Read the model definition and answer for the solid it produces. Units are mm, in the model's axes. A direction names the side the tool comes from. Give positions to 0.01 mm unless a question says otherwise; leave off trailing zeros. Loops run counter-clockwise (first coordinate to the right, second up) from the corner with the lowest first, then second, coordinate; pieces in that order, holes last. Notation, with made-up numbers: (58, 87) - (105, 87) arc R6 ccw to (105, 94) - close; hole circle Ø8 at (35, -12.5). An arc over 180 degrees is marked (long way). Write item = value, one per line. Start each with the question number.
from build123d import *

# Parameters (mm, degrees)
F0_W     = 1333.5
F0_H     = 1524
F0_W_2   = 34.925
F0_H_2   = 63.5
F0_W_3   = 63.5
F0_H_3   = 15.875
F0_W_4   = 15.875
F0_H_4   = 15
F0_H_5   = 95.25
F0_W_5   = 184.15
F0_H_6   = 101.6
F1_DEPTH = 12.7
F2_START = 12.7
F2_DEPTH = 355.6


with BuildPart() as f1:
    # F0 (on Front) → F1 (new body)
    with BuildSketch(Plane.XZ):
        with Locations((666.75, 762)):
            Rectangle(F0_W, F0_H)
        with Locations((166.6875, 39.6875)):
            Rectangle(F0_W_2, F0_H_2, mode=Mode.SUBTRACT)
        with Locations((166.6875, 357.1875)):
            Rectangle(F0_W_2, F0_H_2, mode=Mode.SUBTRACT)
        with Locations((627.0625, 93.6625)):
            Rectangle(F0_W_3, F0_H_3, mode=Mode.SUBTRACT)
        with Locations((627.0625, 279.4)):
            Rectangle(F0_W_3, F0_H_3, mode=Mode.SUBTRACT)
        with Locations((166.6875, 436.5625)):
            Rectangle(F0_W_2, F0_H_2, mode=Mode.SUBTRACT)
        with Locations((92.075, 728.6625)):
            Rectangle(F0_W_4, F0_H_2, mode=Mode.SUBTRACT)
        with Locations((241.3, 728.6625)):
            Rectangle(F0_W_4, F0_H_2, mode=Mode.SUBTRACT)
        with Locations((627.0625, 514.35)):
            Rectangle(F0_W_3, F0_H_3, mode=Mode.SUBTRACT)
        with Locations((627.0625, 650.875)):
            Rectangle(F0_W_3, F0_H_3, mode=Mode.SUBTRACT)
        with Locations((847.725, 39.6875)):
            Rectangle(F0_W_2, F0_H_2, mode=Mode.SUBTRACT)
        with Locations((960.4375, 193.2375)):
            Rectangle(F0_W_3, F0_H_4, mode=Mode.SUBTRACT)
        with Locations((1293.8125, 93.6625)):
            Rectangle(F0_W_3, F0_H_3, mode=Mode.SUBTRACT)
        with Locations((1293.8125, 279.4)):
            Rectangle(F0_W_3, F0_H_3, mode=Mode.SUBTRACT)
        with Locations((847.725, 436.5625)):
            Rectangle(F0_W_2, F0_H_2, mode=Mode.SUBTRACT)
        with Locations((960.4375, 577.85)):
            Rectangle(F0_W_3, F0_H_3, mode=Mode.SUBTRACT)
        with Locations((1293.8125, 514.35)):
            Rectangle(F0_W_3, F0_H_3, mode=Mode.SUBTRACT)
        with Locations((1293.8125, 650.875)):
            Rectangle(F0_W_3, F0_H_3, mode=Mode.SUBTRACT)
        with Locations((25.4, 808.0375)):
            Rectangle(F0_W_2, F0_H_2, mode=Mode.SUBTRACT)
        with Locations((214.3125, 1084.2625)):
            Rectangle(F0_W_4, F0_H_5, mode=Mode.SUBTRACT)
        with Locations((403.225, 808.0375)):
            Rectangle(F0_W_2, F0_H_2, mode=Mode.SUBTRACT)
        with Locations((188.9125, 1179.5125)):
            Rectangle(F0_W_4, F0_H_2, mode=Mode.SUBTRACT)
        with Locations((117.475, 1484.3125)):
            Rectangle(F0_W_4, F0_H_2, mode=Mode.SUBTRACT)
        with Locations((260.35, 1484.3125)):
            Rectangle(F0_W_4, F0_H_2, mode=Mode.SUBTRACT)
        with Locations((617.5375, 1244.6)):
            Rectangle(F0_W_3, F0_H_3, mode=Mode.SUBTRACT)
        with Locations((477.8375, 1406.525)):
            Rectangle(F0_W_5, F0_H_3, mode=Mode.SUBTRACT)
        with Locations((1109.6625, 1081.0875)):
            Rectangle(F0_W_4, F0_H_6, mode=Mode.SUBTRACT)
        with Locations((915.9875, 1419.225)):
            Rectangle(F0_W_3, F0_H_3, mode=Mode.SUBTRACT)
        with Locations((1144.5875, 1179.5125)):
            Rectangle(F0_W_4, F0_H_2, mode=Mode.SUBTRACT)
        with Locations((1144.5875, 1484.3125)):
            Rectangle(F0_W_4, F0_H_2, mode=Mode.SUBTRACT)
        with Locations((477.8375, 1406.525)):
            Rectangle(F0_W_5, F0_H_3)
        with Locations((166.6875, 39.6875)):
            Rectangle(F0_W_2, F0_H_2)
        with Locations((847.725, 39.6875)):
            Rectangle(F0_W_2, F0_H_2)
        with Locations((166.6875, 357.1875)):
            Rectangle(F0_W_2, F0_H_2)
        with Locations((166.6875, 436.5625)):
            Rectangle(F0_W_2, F0_H_2)
        with Locations((847.725, 436.5625)):
            Rectangle(F0_W_2, F0_H_2)
        with Locations((403.225, 808.0375)):
            Rectangle(F0_W_2, F0_H_2)
        with Locations((25.4, 808.0375)):
            Rectangle(F0_W_2, F0_H_2)
        with Locations((1109.6625, 1081.0875)):
            Rectangle(F0_W_4, F0_H_6)
        with Locations((214.3125, 1084.2625)):
            Rectangle(F0_W_4, F0_H_5)
        with Locations((627.0625, 93.6625)):
            Rectangle(F0_W_3, F0_H_3)
        with Locations((627.0625, 279.4)):
            Rectangle(F0_W_3, F0_H_3)
        with Locations((1293.8125, 93.6625)):
            Rectangle(F0_W_3, F0_H_3)
        with Locations((1293.8125, 279.4)):
            Rectangle(F0_W_3, F0_H_3)
        with Locations((627.0625, 514.35)):
            Rectangle(F0_W_3, F0_H_3)
        with Locations((960.4375, 577.85)):
            Rectangle(F0_W_3, F0_H_3)
        with Locations((1293.8125, 514.35)):
            Rectangle(F0_W_3, F0_H_3)
        with Locations((1293.8125, 650.875)):
            Rectangle(F0_W_3, F0_H_3)
        with Locations((627.0625, 650.875)):
            Rectangle(F0_W_3, F0_H_3)
        with Locations((92.075, 728.6625)):
            Rectangle(F0_W_4, F0_H_2)
        with Locations((241.3, 728.6625)):
            Rectangle(F0_W_4, F0_H_2)
        with Locations((188.9125, 1179.5125)):
            Rectangle(F0_W_4, F0_H_2)
        with Locations((117.475, 1484.3125)):
            Rectangle(F0_W_4, F0_H_2)
        with Locations((260.35, 1484.3125)):
            Rectangle(F0_W_4, F0_H_2)
        with Locations((617.5375, 1244.6)):
            Rectangle(F0_W_3, F0_H_3)
        with Locations((915.9875, 1419.225)):
            Rectangle(F0_W_3, F0_H_3)
        with Locations((1144.5875, 1484.3125)):
            Rectangle(F0_W_4, F0_H_2)
        with Locations((1144.5875, 1179.5125)):
            Rectangle(F0_W_4, F0_H_2)
        with Locations((960.4375, 193.2375)):
            Rectangle(F0_W_3, F0_H_4)
    extrude(amount=F1_DEPTH)

    # F0 (on Front) → F2 (join)
    with BuildSketch(Plane.XZ.offset(F2_START)):
        with Locations((1144.5875, 1484.3125)):
            Rectangle(F0_W_4, F0_H_2)
        with Locations((1144.5875, 1179.5125)):
            Rectangle(F0_W_4, F0_H_2)
        with Locations((1109.6625, 1081.0875)):
            Rectangle(F0_W_4, F0_H_6)
        with Locations((915.9875, 1419.225)):
            Rectangle(F0_W_3, F0_H_3)
        with Locations((617.5375, 1244.6)):
            Rectangle(F0_W_3, F0_H_3)
        with Locations((188.9125, 1179.5125)):
            Rectangle(F0_W_4, F0_H_2)
        with Locations((260.35, 1484.3125)):
            Rectangle(F0_W_4, F0_H_2)
        with Locations((117.475, 1484.3125)):
            Rectangle(F0_W_4, F0_H_2)
        with Locations((25.4, 808.0375)):
            Rectangle(F0_W_2, F0_H_2)
        with Locations((214.3125, 1084.2625)):
            Rectangle(F0_W_4, F0_H_5)
        with Locations((403.225, 808.0375)):
            Rectangle(F0_W_2, F0_H_2)
        with Locations((241.3, 728.6625)):
            Rectangle(F0_W_4, F0_H_2)
        with Locations((92.075, 728.6625)):
            Rectangle(F0_W_4, F0_H_2)
        with Locations((166.6875, 436.5625)):
            Rectangle(F0_W_2, F0_H_2)
        with Locations((627.0625, 514.35)):
            Rectangle(F0_W_3, F0_H_3)
        with Locations((627.0625, 650.875)):
            Rectangle(F0_W_3, F0_H_3)
        with Locations((960.4375, 577.85)):
            Rectangle(F0_W_3, F0_H_3)
        with Locations((847.725, 436.5625)):
            Rectangle(F0_W_2, F0_H_2)
        with Locations((1293.8125, 514.35)):
            Rectangle(F0_W_3, F0_H_3)
        with Locations((1293.8125, 650.875)):
            Rectangle(F0_W_3, F0_H_3)
        with Locations((1293.8125, 93.6625)):
            Rectangle(F0_W_3, F0_H_3)
        with Locations((1293.8125, 279.4)):
            Rectangle(F0_W_3, F0_H_3)
        with Locations((960.4375, 193.2375)):
            Rectangle(F0_W_3, F0_H_4)
        with Locations((847.725, 39.6875)):
            Rectangle(F0_W_2, F0_H_2)
        with Locations((627.0625, 93.6625)):
            Rectangle(F0_W_3, F0_H_3)
        with Locations((627.0625, 279.4)):
            Rectangle(F0_W_3, F0_H_3)
        with Locations((166.6875, 39.6875)):
            Rectangle(F0_W_2, F0_H_2)
        with Locations((166.6875, 357.1875)):
            Rectangle(F0_W_2, F0_H_2)
    extrude(amount=F2_DEPTH)


solid = f1.part
1. For a pull along Z with two mould halves and no side action, classify faces 6 (the flat face through (166, -188, 404.812)), 7 (the flat face through (617, -188, 1252.538)), 8 (the flat face through (385.763, -188, 808)) as released by +Z, released by -Z, zero draft, split by the parting line, or undercut.
2. A cutting plane is placed at D-D on z = 1377. Give the vertices of the cut face in (x, y), and give its area (3 significant figures).
3. Given P1, Ø8, axis at y = -276.5, z = 576.5, coming from the -X side; P2, Ø8, axis at x = 1144.5, y = -264, coming from the +Z side; P3, Ø4, axis at x = 314, z = 662.5, coming from the -Y side, each flat-ended and moving along its own axis, determine where each tip first touches the part or whether it passes through.
4. A cutting plane is placed at B-B on z = 1074. Give the vertices of the cut face in (x, y) (3 decimals).
5. Consider line 1 along X through (y, z) = (-186.5, 1187) (3 decimals); line 2 along Z through (x, y) = (596.5, -140) (1 decimal); line 3 along Z through (x, y) = (174.5, -269.5). Determine where each line is inside the solid, lowest interval first. Write a range as [from, to].
6. A cutting plane is placed at C-C on x = 543. Give the vertices of the cut face in (y, z).
7. A tool of negligible diameter and unlimited length cuts with its end or side. For faces 1 (the flat face through (830.262, -188, 436)), 2 (the flat face through (109.538, -188, 1484)), 3 (the flat face through (960, -188, 200.738)), 4 (the flat face through (1152.525, -188, 1484)), 5 (the flat face through (184.15, -188, 357)), from which of +Z, -Z, +X, -X, +Y, -Y can it reach the whole face along a straight path? Write none if from no direction.
8. A cutting plane is placed at A-A on y = -328. Give the number of separate pieces and of enclosed holes in the cut face, and give its area (3 significant figures).
Reply:
q1.face_6 = undercut
q1.face_7 = released by +Z
q1.face_8 = zero draft
q2.outline = (0, -12.7) - (1333.5, -12.7) - (1333.5, 0) - (0, 0) - close
q2.area = 16,900 mm^2
q3.P1 = 928.69
q3.P2 = 1516.06
q3.P3 = -12.7
q4.outline = (0, -12.7) - (206.375, -12.7) - (206.375, -368.3) - (222.25, -368.3) - (222.25, -12.7) - (1101.725, -12.7) - (1101.725, -368.3) - (1117.6, -368.3) - (1117.6, -12.7) - (1333.5, -12.7) - (1333.5, 0) - (0, 0) - close
q5.line_1 = [180.975, 196.85], [1136.65, 1152.525]
q5.line_2 = [85.7, 101.6], [271.5, 287.3], [506.4, 522.3], [642.9, 658.8], [1236.7, 1252.5]
q5.line_3 = [7.94, 71.44], [325.44, 388.94], [404.81, 468.31]
q6.outline = (-12.7, 0) - (0, 0) - (0, 1524) - (-12.7, 1524) - close
q7.face_1 = +Z, -Z, -Y
q7.face_2 = +Z, -Z, -X, -Y
q7.face_3 = +X, -X, -Y
q7.face_4 = +Z, -Z, +X, -Y
q7.face_5 = -Z, +X, -Y
q8.separate_pieces = 28
q8.enclosed_holes = 0
q8.area = 37,700 mm^2
